Part model, mm, in its own coordinate system. A direction names the side the tool comes from. Give positions to 0.01 mm unless a question says otherwise; leave off trailing zeros. Order: outer loops, then holes, each group sorted by start corner. A loop starts at its lowest first (then second) coordinate and runs counter-clockwise, first axis right, second up. Notation, with made-up numbers: (22.5, 72.5) - (50.5, 72.5) arc R16 ccw to (50.5, 81.5) - close; hole circle Ø2 at (23.25, 81). An arc over 180 degrees is marked (long way). Use a Markdown table: item, result. Add a question column.
from build123d import *

# Parameters (mm, degrees)
SKETCH1_W           = 1300
SKETCH1_H           = 700
BOSS_EXTRUDE1_DEPTH = 150
SKETCH2_W           = 1050
SKETCH2_H           = 550
CUT_EXTRUDE1_DEPTH  = 50
SKETCH3_W           = 1050
SKETCH3_H           = 550
CUT_EXTRUDE2_DEPTH  = 50
SKETCH14_W          = 100
SKETCH14_H          = 80
BOSS_EXTRUDE3_DEPTH = 60
SKETCH15_W          = 93
SKETCH15_H          = 55
CUT_EXTRUDE7_DEPTH  = 40
SKETCH16_W          = 100
SKETCH16_H          = 80
BOSS_EXTRUDE4_DEPTH = 60


with BuildPart() as part:
    # Sketch1 → Boss-Extrude1 (new body)
    with BuildSketch(Plane(origin=(0, 0, 0), x_dir=(1, 0, 0), z_dir=(0, 1, 0))):
        Rectangle(SKETCH1_W, SKETCH1_H)
    extrude(amount=BOSS_EXTRUDE1_DEPTH)

    # Sketch2 → Cut-Extrude1 (cut)
    with BuildSketch(Plane(origin=(0, 150, 0), x_dir=(1, 0, 0), z_dir=(0, 1, 0))):
        Rectangle(SKETCH2_W, SKETCH2_H)
    extrude(amount=-CUT_EXTRUDE1_DEPTH, mode=Mode.SUBTRACT)

    # Sketch3 → Cut-Extrude2 (cut)
    with BuildSketch(Plane.XZ):
        Rectangle(SKETCH3_W, SKETCH3_H)
    extrude(amount=-CUT_EXTRUDE2_DEPTH, mode=Mode.SUBTRACT)

    # Sketch14 → Boss-Extrude3 (add)
    with BuildSketch(Plane(origin=(0, 150, 0), x_dir=(1, 0, 0), z_dir=(0, 1, 0))):
        with Locations((485, -390)):
            Rectangle(SKETCH14_W, SKETCH14_H)
        with Locations((-485, -390)):
            Rectangle(SKETCH14_W, SKETCH14_H)
    extrude(amount=-BOSS_EXTRUDE3_DEPTH)

    # Sketch15 → Cut-Extrude7 (cut)
    with BuildSketch(Plane.XZ.offset(-90)):
        with Locations((485.587200579, 389.924483471)):
            Rectangle(SKETCH15_W, SKETCH15_H)
    extrude(amount=-CUT_EXTRUDE7_DEPTH, mode=Mode.SUBTRACT)

    # Sketch16 → Boss-Extrude4 (add)
    with BuildSketch(Plane(origin=(0, 150, 0), x_dir=(1, 0, 0), z_dir=(0, 1, 0))):
        with Locations((485, 390)):
            Rectangle(SKETCH16_W, SKETCH16_H)
        with Locations((-485, 390)):
            Rectangle(SKETCH16_W, SKETCH16_H)
    extrude(amount=-BOSS_EXTRUDE4_DEPTH)


solid = part.part
1. Cut at D-D (x = 551.5). Write the cut outline in (y, z), plus the area to 3 significant figures.
2. Cut at B-B (z = 198). Write the cut outline in (x, y), plus the area to 3 significant figures.
3. Tool access for faces 4 (the face through (435, 120, -389)), 5 (the face through (485, 130, 390)), 6 (the face through (484, 90, -391)): list every direction of +Z, -Z, +X, -X, +Y, -Y with a clear straight run to the whole face (end or side of a thin tool).
4. Drill centre lines: probe 1 along Z at (x, y) = (282, 35); probe 2 along X at (y, z) = (115.5, 154.5); probe 3 along Z at (x, y) = (25, 90.5). Where is each one in solid material? Low to high. Write a range as [from, to].
5. Mould opens along Z. For faces 1 (the face through (439.087, 110, 390)), 2 (the face through (-435, 120, 391)), 3 (the face through (484, 120, 430)) say: released by +Z, released by -Z, zero draft, split by the parting line, or undercut.
6. Cut at C-C (x = 126). Write the cut outline in (y, z).
7. Pin check, flat tips, straight feed: P1, Ø1.5, axis at x = 376.5, y = 99.5, coming from the +Z side; P2, Ø18, axis at y = 117.5, z = 380.5, coming from the -X side; P3, Ø24, axis at x = 501, z = -395, coming from the -Y side. Stop position of each tip, or through.
8. Cut at A-A (y = 21). Write the cut outline in (x, z), plus the area to 4 significant figures.
Responses:
| question | item | result |
|---|---|---|
| 1 | outline | (0, -350) - (150, -350) - (150, 350) - (0, 350) - close |
| 1 | area | 105,000 mm² |
| 2 | outline | (-650, 0) - (-525, 0) - (-525, 50) - (525, 50) - (525, 0) - (650, 0) - (650, 150) - (525, 150) - (525, 100) - (-525, 100) - (-525, 150) - (-650, 150) - close |
| 2 | area | 90,000 mm² |
| 3 | face 4 | -Z, +Y, -Y |
| 3 | face 5 | -Y |
| 3 | face 6 | -Z, +X, -X, -Y |
| 4 | probe 1 | z = [-350, -275], [275, 350] |
| 4 | probe 2 | x = [-650, -525], [525, 650] |
| 4 | probe 3 | z = [-350, 350] |
| 5 | face 1 | undercut |
| 5 | face 2 | zero draft |
| 5 | face 3 | released by +Z |
| 6 | outline | (0, -350) - (150, -350) - (150, -275) - (100, -275) - (100, 275) - (150, 275) - (150, 350) - (0, 350) - (0, 275) - (50, 275) - (50, -275) - (0, -275) - close |
| 7 | P1 | stops at z = 350 |
| 7 | P2 | stops at x = -535 |
| 7 | P3 | stops at y = 90 |
| 8 | outline | (-650, -350) - (650, -350) - (650, 350) - (-650, 350) - close; hole (-525, -275) - (525, -275) - (525, 275) - (-525, 275) - close |
| 8 | area | 332,500 mm² |
